The listing builds one solid part. Answer for the finished solid, in the listing's coordinates (mm). Face numbers are marked on the shaded views. A direction names the side the tool comes from. Round coordinates to 2 decimals unless told otherwise and drop trailing zeros. Order: outer loops, then holes, each group sorted by start corner. A loop starts at its lowest first (then second) coordinate and runs counter-clockwise, first axis right, second up. Notation, with made-up numbers: (77, -14) -> (123, -14) arc R20 cw to (123, 14) -> close; hole circle Ø6 at (62, -38.75). An arc over 180 degrees is marked (long way). Answer in a Markdown table with one row per item. Add a question column.
```python
from build123d import *

# Parameters (mm, degrees)
SKETCH_R     = 8
PAD_DEPTH    = 5
PAD001_DEPTH = 20


with BuildPart() as part:
    # Sketch → Pad (new body)
    with BuildSketch(Plane.XY):
        with BuildLine():
            ThreePointArc((-2.4, -9.707729), (10, 0), (-2.4, 9.707729))
            Line((-25.96, 3.883092), (-2.4, 9.707729))
            ThreePointArc((-25.96, 3.883092), (-29, 0), (-25.96, -3.883092))
            Line((-2.4, -9.707729), (-25.96, -3.883092))
        make_face()
        Circle(SKETCH_R, mode=Mode.SUBTRACT)
    extrude(amount=PAD_DEPTH)

    # Sketch001 (on Face7 of Pad) → Pad001 (join)
    with BuildSketch(Plane.XY.offset(5)):
        with BuildLine():
            ThreePointArc((-25.96, 3.883092), (-29, 0), (-25.96, -3.883092))
            Line((-21, -5.109331), (-25.96, -3.883092))
            Line((-21, -5.109331), (-21, 5.109331))
            Line((-21, 5.109331), (-25.96, 3.883092))
        make_face()
    extrude(amount=PAD001_DEPTH)


solid = part.part
```
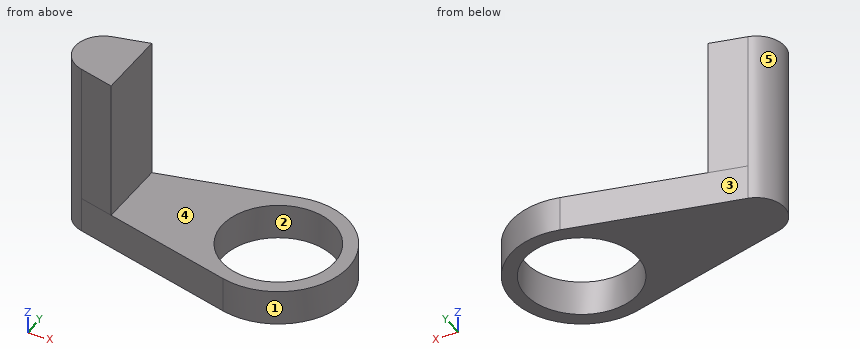
Item 1: Find the intervals of material crossed by probe 1 along Y at (x, z) = (0, 3.3); probe 2 along Z at (x, y) = (7, -6.5); probe 3 along Y at (x, z) = (-17, 1.5), in increasing order. Write a range as [from, to].
Item 2: A tool of negligible diameter and unlimited length cuts with its end or side. For the marked faces 4 and 5, from which of +Z, -Z, +X, -X, +Y, -Y can it reach the whole face along a straight path? Write none if from no direction.
Item 3: The part is cut by section A-A, the plane y = 0. Give the vertices of the cut face in (x, z), and give its area (3 significant figures).
Item 4: The part is cut by section D-D, the plane x = 5.5. Give the vertices of the cut face in (y, z), and give its area (3 significant figures).
Item 5: Flat-ended cylindrical pins translate along their axes: P1, Ø6, axis at x = -12.5, y = -1, coming from the +Z side; P2, Ø5, axis at x = 2.5, y = -5, coming from the -Z side; P3, Ø2, axis at x = -21.5, z = 21.5, coming from the +Y side; P4, Ø3, axis at y = 1.5, z = 11, coming from the +X side. Find the tip coordinate at first contact, or state that the pin passes through.
Item 6: The part is cut by section C-C, the plane z = 19.5. Give the vertices of the cut face in (x, y), and give its area (3 significant figures).
Item 7: The part is cut by section B-B, the plane x = 0. Give the vertices of the cut face in (y, z).
Item 8: For a pull along X with two mould halves and no side action, classify the marked faces 1, 2 and 3 as released by +X, released by -X, zero draft, split by the parting line, or undercut.
Resolved:
| question | item | result |
|---|---|---|
| 1 | probe 1 | [-10, -8], [8, 10] |
| 1 | probe 2 | [0, 5] |
| 1 | probe 3 | [-6.1, 6.1] |
| 2 | face 4 | +Z, +X, +Y, -Y |
| 2 | face 5 | +Z, -Z, -X |
| 3 | outline | (-29, 0) -> (-8, 0) -> (-8, 5) -> (-21, 5) -> (-21, 25) -> (-29, 25) -> close; (8, 0) -> (10, 0) -> (10, 5) -> (8, 5) -> close |
| 3 | area | 275 mm2 |
| 4 | outline | (-8.35, 0) -> (-5.81, 0) -> (-5.81, 5) -> (-8.35, 5) -> close; (5.81, 0) -> (8.35, 0) -> (8.35, 5) -> (5.81, 5) -> close |
| 4 | area | 25.4 mm2 |
| 5 | P1 | z = 5 |
| 5 | P2 | z = 0 |
| 5 | P3 | y = 5.11 |
| 5 | P4 | x = -21 |
| 6 | outline | (-25.96, -3.88) -> (-21, -5.11) -> (-21, 5.11) -> (-25.96, 3.88) arc R4 ccw to start |
| 6 | area | 62.1 mm2 |
| 7 | outline | (-10, 0) -> (-8, 0) -> (-8, 5) -> (-10, 5) -> close; (8, 0) -> (10, 0) -> (10, 5) -> (8, 5) -> close |
| 8 | face 1 | split by the parting line |
| 8 | face 2 | undercut |
| 8 | face 3 | released by -X |
